```python
from build123d import *

# Parameters (mm, degrees)
SKETCH1_R           = 1.875
BOSS_EXTRUDE1_DEPTH = 2


with BuildPart() as part:
    # Sketch1 → Boss-Extrude1 (new body)
    with BuildSketch(Plane.XY):
        with BuildLine():
            Line((0, 4.5), (60, 4.5))
            ThreePointArc((60, 4.5), (63.63873393, -2.647567824), (55.718313389, -1.384615385))
            ThreePointArc((55.718313389, -1.384615385), (54.992038372, -0.38278492), (53.815341562, 0))
            Line((53.815341562, 0), (6.184658438, 0))
            ThreePointArc((6.184658438, 0), (5.007961628, -0.38278492), (4.281686611, -1.384615385))
            ThreePointArc((4.281686611, -1.384615385), (-3.63873393, -2.647567824), (0, 4.5))
        make_face()
        Circle(SKETCH1_R, mode=Mode.SUBTRACT)
        with Locations((60, 0)):
            Circle(SKETCH1_R, mode=Mode.SUBTRACT)
    extrude(amount=BOSS_EXTRUDE1_DEPTH)


solid = part.part
```
Verification items for the finished model (mm, model axes). A direction names the side the tool comes from. Round coordinates to 2 decimals unless told otherwise and drop trailing zeros. Write each loop counter-clockwise with the first axis right and the second up, starting at its lowest first coordinate (ties: lowest second). Pieces come first, ordered by that corner, then holes. Notation, with made-up numbers: (3, 8.5) - (36, 8.5) arc R21 cw to (36, 38.5) - close; hole circle Ø6 at (84, 41). An arc over 180 degrees is marked (long way). Answer as a JSON object with one key per item and string values. Group by question number.
Q1. Section check C-C, the plane y = 3. Enter the section's corners in (x, z).
Q2. Section check A-A, the plane z = 0.85. Enter the section's corners in (x, y) (3 decimals), plus the area to 3 significant figures.
Q3. Tool access check on faces 1 (the cylindrical face through (63.72, -2.53, 0.99)), 2 (the cylindrical face through (5.022, -0.372, 0.986)). Record the directions out of +Z, -Z, +X, -X, +Y, -Y that give a thin tool (end or side, any length) a straight path to the whole face; none if there is none.
Q4. Section check B-B, the plane x = 25. Enter the section's corners in (y, z).
Q5. Mould release check, pull along Y, two halves, no side actions. Record for faces 3 (the cylindrical face through (58.51, -1.14, 0.99)), 4 (the flat face through (30, 0, 1)), 5 (the flat face through (30, 1, 2)): released by +Y, released by -Y, zero draft, split by the parting line, or undercut.
Q6. Thickness scan on line 1 (Y direction, x = 0, z = 1.2) (3 decimals); line 2 (X direction, y = -3, z = 1.55); line 3 (X direction, y = 1.5, z = 1.15) (3 decimals). Record the ranges inside material, lowest first.
Found:
{
 "1": {"outline": "(-3.35, 0) - (63.35, 0) - (63.35, 2) - (-3.35, 2) - close"},
 "2": {"outline": "(0, 4.5) arc R4.5 ccw (long way) to (4.282, -1.385) arc R2 cw to (6.185, 0) - (53.815, 0) arc R2 cw to (55.718, -1.385) arc R4.5 ccw (long way) to (60, 4.5) - close; hole circle Ø3.75 at (0, 0); hole circle Ø3.75 at (60, 0)", "area": "344 mm^2"},
 "3": {"face 1": "+Z, -Z", "face 2": "+Z, -Z, -Y"},
 "4": {"outline": "(0, 0) - (4.5, 0) - (4.5, 2) - (0, 2) - close"},
 "5": {"face 3": "undercut", "face 4": "released by -Y", "face 5": "zero draft"},
 "6": {"line 1": "y = -4.5 to -1.875, 1.875 to 4.5", "line 2": "x = -3.35 to 3.35, 56.65 to 63.35", "line 3": "x = -4.243 to -1.125, 1.125 to 58.875, 61.125 to 64.243"}
}
